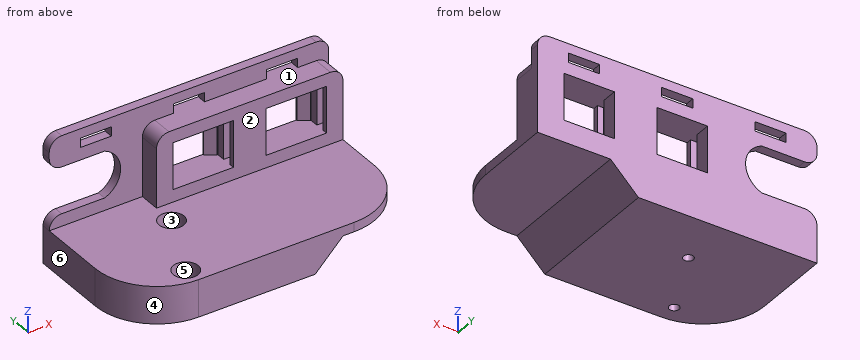
```python
from build123d import *

# Parameters (mm, degrees)
SKETCH_W        = 90
SKETCH_H        = 45
PAD_DEPTH       = 16
POCKET_DEPTH    = 60
PAD001_DEPTH    = 15
POCKET001_DEPTH = 4
PAD002_DEPTH    = 4
POCKET002_DEPTH = 5
SKETCH006_W     = 90
SKETCH006_H     = 3
PAD003_DEPTH    = 6
SKETCH007_W     = 10
SKETCH007_H     = 3
POCKET003_DEPTH = 5
SKETCH008_R     = 1.6
POCKET004_DEPTH = 20
SKETCH009_R     = 4
POCKET005_DEPTH = 8
FILLET_R        = 4
FILLET001_R     = 4
FILLET002_R     = 20
SKETCH010_W     = 18.432236
SKETCH010_H     = 15
POCKET006_DEPTH = 5
FILLET003_R     = 4
CHAMFER_1_SIZE2 = 3
CHAMFER_1_SIZE  = 2
CHAMFER_2_SIZE2 = 3
CHAMFER_2_SIZE  = 2


with BuildPart() as part:
    # Sketch → Pad (new body)
    with BuildSketch(Plane.XY):
        with Locations((15, -5.5)):
            Rectangle(SKETCH_W, SKETCH_H)
    extrude(amount=PAD_DEPTH)

    # Sketch001 (on Face2 of Pad) → Pocket (cut)
    with BuildSketch(Plane.XZ.offset(28)):
        Polygon((60, 0), (60, 9), (36.5, 9), (27.5, 0), align=None)
    extrude(amount=-POCKET_DEPTH, mode=Mode.SUBTRACT)

    # Sketch002 (on Face5 of Pocket) → Pad001 (join)
    with BuildSketch(Plane.XY.offset(16)):
        Polygon((54.75, 7.2), (54.75, 8.9), (56.75, 8.9), (56.75, 11.9), (54.75, 11.9), (54.75, 14.7), (51.55, 14.7), (51.55, 17), (60, 17), (60, 7.2), align=None)
        Polygon((35.25, 7.2), (35.25, 8.9), (33.25, 8.9), (33.25, 11.9), (35.25, 11.9), (35.25, 17), (21.55, 17), (21.55, 14.7), (24.75, 14.7), (24.75, 11.9), (26.75, 11.9), (26.75, 8.9), (24.75, 8.9), (24.75, 7.2), align=None)
        Polygon((5.25, 7.2), (5.25, 8.9), (3.25, 8.9), (3.25, 11.9), (5.25, 11.9), (5.25, 17), (-30, 17), (-30, 14), (0, 14), (0, 7.2), align=None)
    extrude(amount=PAD001_DEPTH)

    # Sketch003 (on Face3 of Pad001) → Pocket001 (cut)
    with BuildSketch(Plane.XY.offset(16)):
        Polygon((-30, -28), (-30, 14), (0, 14), (0, 7.2), (60, 7.2), (60, -28), align=None)
    extrude(amount=-POCKET001_DEPTH, mode=Mode.SUBTRACT)

    # Sketch004 (on Face9 of Pocket001) → Pad002 (join)
    with BuildSketch(Plane.XY.offset(31)):
        Polygon((-30, 17), (60, 17), (60, 7.2), (0, 7.2), (0, 14), (-30, 14), align=None)
    extrude(amount=PAD002_DEPTH)

    # Sketch005 (on Face39 of Pad002) → Pocket002 (cut)
    with BuildSketch(Plane.XZ.offset(-14)):
        with BuildLine():
            ThreePointArc((-12.216118, 16), (-7, 23.5), (-12.216118, 31))
            Line((-12.216118, 31), (-17.783882, 31))
            ThreePointArc((-17.783882, 31), (-23, 23.5), (-17.783882, 16))
            Line((-17.783882, 16), (-12.216118, 16))
        make_face()
    extrude(amount=-POCKET002_DEPTH, mode=Mode.SUBTRACT)

    # Sketch006 (on Face9 of Pocket002) → Pad003 (join)
    with BuildSketch(Plane.XY.offset(35)):
        with Locations((15, 15.5)):
            Rectangle(SKETCH006_W, SKETCH006_H)
    extrude(amount=PAD003_DEPTH)

    # Sketch007 (on Face45 of Pad003) → Pocket003 (cut)
    with BuildSketch(Plane.XZ.offset(-14)):
        with Locations((-15, 36.5)):
            Rectangle(SKETCH007_W, SKETCH007_H)
        with Locations((15, 36.5)):
            Rectangle(SKETCH007_W, SKETCH007_H)
        with Locations((45, 36.5)):
            Rectangle(SKETCH007_W, SKETCH007_H)
    extrude(amount=-POCKET003_DEPTH, mode=Mode.SUBTRACT)

    # Sketch008 (on Face43 of Pocket003) → Pocket004 (cut)
    with BuildSketch(Plane.XY.offset(12)):
        Circle(SKETCH008_R)
        with Locations((-10.3, -22.2)):
            Circle(SKETCH008_R)
    extrude(amount=-POCKET004_DEPTH, mode=Mode.SUBTRACT)

    # Sketch009 (on Face44 of Pocket004) → Pocket005 (cut)
    with BuildSketch(Plane.XY.offset(12)):
        with Locations((-10.3, -22.2)):
            Circle(SKETCH009_R)
        Circle(SKETCH009_R)
    extrude(amount=-POCKET005_DEPTH, mode=Mode.SUBTRACT)

    # Fillet
    fillet_edges = [part.edges().sort_by_distance(p)[0] for p in [
        (-30, 15.5, 41),
        (60, 15.5, 41),
    ]]
    fillet(fillet_edges, radius=FILLET_R)

    # Fillet001
    fillet001_edges = [part.edges().sort_by_distance(p)[0] for p in [
        (60, 10.6, 35),
        (0, 10.6, 35),
    ]]
    fillet(fillet001_edges, radius=FILLET001_R)

    # Fillet002
    fillet002_edges = [part.edges().sort_by_distance(p)[0] for p in [
        (-30, -28, 6),
        (60, -28, 10.5),
    ]]
    fillet(fillet002_edges, radius=FILLET002_R)

    # Sketch010 (on Face8 of Fillet002) → Pocket006 (cut)
    with BuildSketch(Plane.XZ.offset(-14)):
        with Locations((-27, 23.5)):
            Rectangle(SKETCH010_W, SKETCH010_H)
    extrude(amount=-POCKET006_DEPTH, mode=Mode.SUBTRACT)

    # Fillet003
    fillet003_edges = [part.edges().sort_by_distance(p)[0] for p in [
        (-30, 15.5, 31),
        (-30, 15.5, 16),
    ]]
    fillet(fillet003_edges, radius=FILLET003_R)

    # Chamfer 1
    chamfer_1_edges = [part.edges().sort_by_distance(p)[0] for p in [
        (21.55, 14.7, 23.5),
    ]]
    chamfer_1_side = part.faces().sort_by_distance((21.55, 15.85, 23.5))[0]
    chamfer(chamfer_1_edges, length=CHAMFER_1_SIZE, length2=CHAMFER_1_SIZE2, reference=chamfer_1_side)

    # Chamfer 2
    chamfer_2_edges = [part.edges().sort_by_distance(p)[0] for p in [
        (51.55, 14.7, 23.5),
    ]]
    chamfer_2_side = part.faces().sort_by_distance((51.55, 15.85, 23.5))[0]
    chamfer(chamfer_2_edges, length=CHAMFER_2_SIZE, length2=CHAMFER_2_SIZE2, reference=chamfer_2_side)


solid = part.part
```
CAD build for the part. Positions are in the model's coordinates, mm. Face numbers are marked on the shaded views. A direction names the side the tool comes from. Give positions to 0.01 mm unless a question says otherwise; leave off trailing zeros. Write each loop counter-clockwise with the first axis right and the second up, starting at its lowest first coordinate (ties: lowest second). Pieces come first, ordered by that corner, then holes. Notation, with made-up numbers: M -10,60 L 13,60 A5 ccw 13,64 Z; hole C -2,-37.75 d1. An arc over 180 degrees is marked long. Return JSON: item names as keys, results as strings. Group by question number.
(1) Drill centre lines: L1, parallel to Z at x = 15.5, y = 10; L2, parallel to X at y = 9, z = 30.5; L3, parallel to Y at x = 0, z = 7. Where is each one in solid material? Low to high. Write a range as [from, to].
(2) Mould opens along Y. For the marked faces 4, 5 and 6 say: pulls with the +Y half, pulls with the -Y half, needs draft (parallel to the pull), parting line crosses it, or undercut.
(3) Band-saw the part on C-C (y = 0). Give the cut face in (x, z).
(4) 3-axis set-ups, long thin cutter, end or side, ignore diameter. For the marked faces 1, 2 and 3: which of +Z, -Z, +X, -X, +Y, -Y reach the whole face in a straight line?
(5) Flat gauge pins, fed straight in: pin 1 Ø1.6 at (x, z) = (4.5, 26) entering from -Y; pin 2 Ø3 at (x, y) = (49, 11.5) entering from +Z; pin 3 Ø3 at (y, z) = (14, 20) entering from -X (3 decimals). Where does each tip first touch, or does it go through?
(6) Band-saw the part on A-A (z = 36). Give the cut face in (x, y).
(7) Band-saw the part on D-D (y = 10.5). Give the cut face in (x, z), and give its area (3 significant figures).
(8) Band-saw the part on B-B (x = 12.5). Give the cut face in (y, z).
Entries:
{
 "1": {"L1": "z = [0, 16], [31, 35]", "L2": "x = [0, 3.25], [26.75, 33.25], [56.75, 60]", "L3": "y = [-28, -4], [4, 17]"},
 "2": {"face 4": "pulls with the -Y half", "face 5": "undercut", "face 6": "needs draft"},
 "3": {"outline": "M -30,0 L -1.6,0 L -1.6,4 L -4,4 L -4,12 L -30,12 Z; M 1.6,0 L 27.5,0 L 36.5,9 L 60,9 L 60,12 L 4,12 L 4,4 L 1.6,4 Z"},
 "4": {"face 1": "-Y", "face 2": "+Z, +X, -X, -Y", "face 3": "+Z"},
 "5": {"pin 1": "stops at y = 7.2", "pin 2": "stops at z = 35", "pin 3": "stops at x = -8.755"},
 "6": {"outline": "M -30,14 L -20,14 L -20,17 L -30,17 Z; M -10,14 L 10,14 L 10,17 L -10,17 Z; M 20,14 L 40,14 L 40,17 L 20,17 Z; M 50,14 L 60,14 L 60,17 L 50,17 Z"},
 "7": {"outline": "M -30,0 L 27.5,0 L 36.5,9 L 60,9 L 60,31 A4 ccw 56,35 L 4,35 A4 ccw 0,31 L 0,12 L -30,12 Z; hole M 3.25,16 L 26.75,16 L 26.75,31 L 3.25,31 Z; hole M 33.25,16 L 56.75,16 L 56.75,31 L 33.25,31 Z", "area": "1,500 mm^2"},
 "8": {"outline": "M -28,0 L 17,0 L 17,16 L 7.2,16 L 7.2,12 L -28,12 Z; M 7.2,31 L 17,31 L 17,35 L 7.2,35 Z; M 14,38 L 17,38 L 17,41 L 14,41 Z"}
}
